Design review of the part built by this model. Coordinates are the model's own, in mm. A direction names the side the tool comes from. Give positions to 0.01 mm unless a question says otherwise; leave off trailing zeros. Loops run counter-clockwise (first coordinate to the right, second up) from the corner with the lowest first, then second, coordinate; pieces in that order, holes last. Notation, with made-up numbers: (35, 58) -> (63, 58) arc R25 ccw to (63, 77) -> close; hole circle Ø1 at (37, 37.5). An arc over 180 degrees is marked (long way). Use a Markdown table: item, result. Add a question column.
1. Draft analysis for pull direction Z (two halves, no side actions). For faces 6 (the cylindrical face through (153.73, 74.99, -0.36)), 7 (the cylindrical face through (173.43, 54.89, 4.93)), 8 (the cylindrical face through (73.547, 25.984, -58.915)), state which applies: pulls with the +Z half, pulls with the -Z half, needs draft (parallel to the pull), parting line crosses it, or undercut.
2. For faces 1 (the cylindrical face through (117.019, 12.777, 9.145)), 2 (the cylindrical face through (117.019, 12.777, 0.855)), 3 (the flat face through (116.117, 12, 5)), 4 (the flat face through (142, 33, 0)), 5 (the cylindrical face through (73.547, 47.054, -48.879)), list the 3-axis set-ups (+Z, -Z, +X, -X, +Y, -Y) from which the entire face can be reached by the end or side of a thin tool; tool diameter is ignored.
3. To check wall thickness, follow line 1 (Y direction, x = 113.5, z = -25.5); line 2 (X direction, y = 60.5, z = -61); line 3 (Y direction, x = 78, z = -43). State the ranges of each line that lie inside material, in increasing order.
4. Add section D-D (x = 188.5). State the section outline as (y, z) points.
5. For pin 1 Ø6.5 at (x, y) = (155.62, 56.56) entering from -Z; pin 2 Ø1 at (y, z) = (67, -44.5) entering from +X; pin 3 Ø3 at (y, z) = (15.5, 4) entering from +X, all flat-tipped, find the tip position at first contact; note any pin that passes through.
6. Add section C-C (z = -15.5). State the section outline as (x, y) points, and give its area (3 significant figures).
7. Add section B-B (x = 107.5). State the section outline as (y, z) points.
8. Add section A-A (z = -40). State the section outline as (x, y) points, and give its area (3 significant figures).
```python
from build123d import *

# Parameters (mm, degrees)
SKETCH3_R           = 7.5
SKETCH3_R_2         = 2.75
BOSS_EXTRUDE1_DEPTH = 10
SKETCH4_W           = 10
SKETCH4_H           = 95
BOSS_EXTRUDE2_DEPTH = 70
SKETCH8_R           = 7.5
SKETCH8_R_2         = 2.75
CUT_EXTRUDE2_DEPTH  = 43.8
BOSS_EXTRUDE3_DEPTH = 10
FILLET1_R           = 5
SKETCH11_W          = 25
SKETCH11_H          = 25
CUT_EXTRUDE3_DEPTH  = 11
FILLET3_R           = 3


with BuildPart() as part:
    # Sketch3 → Boss-Extrude1 (new body)
    with BuildSketch(Plane.XY):
        with BuildLine():
            Line((68.617133813, 80.05993294), (163.617133813, 80.05993294))
            ThreePointArc((163.617133813, 80.05993294), (191.90140506, 68.344204188), (203.617133813, 40.05993294))
            Line((203.617133813, 40.05993294), (203.617133813, 25.05993294))
            ThreePointArc((203.617133813, 25.05993294), (191.90140506, -3.224338307), (163.617133813, -14.94006706))
            Line((163.617133813, -14.94006706), (68.617133813, -14.94006706))
            Line((68.617133813, -14.94006706), (68.617133813, 80.05993294))
        make_face()
        with Locations((163.617133813, 32.55993294)):
            Circle(SKETCH3_R, mode=Mode.SUBTRACT)
        with Locations((189.617133813, 42.55993294)):
            Circle(SKETCH3_R_2, mode=Mode.SUBTRACT)
        with Locations((155.617133813, 56.55993294)):
            Circle(SKETCH3_R_2, mode=Mode.SUBTRACT)
        with Locations((175.617133813, 56.55993294)):
            Circle(SKETCH3_R_2, mode=Mode.SUBTRACT)
        with Locations((155.617133813, 8.55993294)):
            Circle(SKETCH3_R_2, mode=Mode.SUBTRACT)
        with Locations((175.617133813, 8.55993294)):
            Circle(SKETCH3_R_2, mode=Mode.SUBTRACT)
        with Locations((189.617133813, 22.55993294)):
            Circle(SKETCH3_R_2, mode=Mode.SUBTRACT)
    extrude(amount=BOSS_EXTRUDE1_DEPTH)

    # Sketch4 → Boss-Extrude2 (add)
    with BuildSketch(Plane(origin=(0, 0, 0), x_dir=(-1, 0, 0), z_dir=(0, 0, -1))):
        with Locations((-73.617133813, 32.55993294)):
            Rectangle(SKETCH4_W, SKETCH4_H)
    extrude(amount=BOSS_EXTRUDE2_DEPTH)

    # Sketch8 → Cut-Extrude2 (cut)
    with BuildSketch(Plane.ZY.offset(-68.617133813)):
        with Locations((-40, 32.55993294)):
            Circle(SKETCH8_R)
        with Locations((-56.167891819, 25.862972874)):
            Circle(SKETCH8_R_2)
        with Locations((-56.167891819, 39.256893006)):
            Circle(SKETCH8_R_2)
        with Locations((-46.696960066, 48.727824759)):
            Circle(SKETCH8_R_2)
        with Locations((-33.303039934, 48.727824759)):
            Circle(SKETCH8_R_2)
        with Locations((-23.832108181, 39.256893006)):
            Circle(SKETCH8_R_2)
        with Locations((-23.832108181, 25.862972874)):
            Circle(SKETCH8_R_2)
        with Locations((-33.303039934, 16.392041121)):
            Circle(SKETCH8_R_2)
        with Locations((-46.696960066, 16.392041121)):
            Circle(SKETCH8_R_2)
    extrude(amount=-CUT_EXTRUDE2_DEPTH, mode=Mode.SUBTRACT)

    # Sketch9 → Boss-Extrude3 (add)
    with BuildSketch(Plane.XZ.offset(14.94006706)):
        Polygon((78.617133813, -70), (153.617133813, 0), (78.617133813, 0), align=None)
    boss_extrude3 = extrude(amount=-BOSS_EXTRUDE3_DEPTH)

    # Mirror1: Boss-Extrude3 across plane
    add(boss_extrude3.mirror(Plane(origin=(0, 32.55993294, 0), x_dir=(0, 0, 1), z_dir=(0, -1, 0))))

    # Fillet1
    fillet1_edges = [part.edges().sort_by_distance(p)[0] for p in [
        (153.617133813, -9.94006706, 0),
        (153.617133813, 75.05993294, 0),
    ]]
    fillet(fillet1_edges, radius=FILLET1_R)

    # Sketch11 → Cut-Extrude3 (cut, through all)
    with BuildSketch(Plane(origin=(0, 0, 0), x_dir=(-1, 0, 0), z_dir=(0, 0, -1))):
        with Locations((-103.617133813, 12.55993294)):
            Rectangle(SKETCH11_W, SKETCH11_H)
    extrude(amount=-CUT_EXTRUDE3_DEPTH, mode=Mode.SUBTRACT)

    # Fillet3
    fillet3_edges = [part.edges().sort_by_distance(p)[0] for p in [
        (91.117133813, 12.55993294, 10),
        (103.617133813, 0.05993294, 10),
        (116.117133813, 12.55993294, 10),
        (103.617133813, 25.05993294, 10),
        (91.117133813, 12.55993294, 0),
        (103.617133813, 25.05993294, 0),
        (116.117133813, 12.55993294, 0),
        (103.617133813, 0.05993294, 0),
    ]]
    fillet(fillet3_edges, radius=FILLET3_R)


solid = part.part
```
Taken from the geometry:
| question | item | result |
|---|---|---|
| 1 | face 6 | pulls with the -Z half |
| 1 | face 7 | needs draft |
| 1 | face 8 | undercut |
| 2 | face 1 | +Z |
| 2 | face 2 | -Z |
| 2 | face 3 | +Z, -Z |
| 2 | face 4 | -Z, +X |
| 2 | face 5 | +X, -X |
| 3 | line 1 | y = -14.94 to -4.94, 70.06 to 80.06 |
| 3 | line 2 | x = 68.62 to 78.62 |
| 3 | line 3 | y = -14.94 to 25.69, 39.43 to 80.06 |
| 4 | outline | (-6.26, 0) -> (20.05, 0) -> (20.05, 10) -> (-6.26, 10) -> close; (25.07, 0) -> (40.05, 0) -> (40.05, 10) -> (25.07, 10) -> close; (45.07, 0) -> (71.38, 0) -> (71.38, 10) -> (45.07, 10) -> close |
| 5 | pin 1 | stops at z = 0 |
| 5 | pin 2 | stops at x = 78.62 |
| 5 | pin 3 | stops at x = 202.8 |
| 6 | outline | (68.62, -14.94) -> (137.01, -14.94) -> (137.01, -4.94) -> (78.62, -4.94) -> (78.62, 70.06) -> (137.01, 70.06) -> (137.01, 80.06) -> (68.62, 80.06) -> close |
| 6 | area | 2,120 mm^2 |
| 7 | outline | (-14.94, -43.04) -> (-4.94, -43.04) -> (-4.94, 0) -> (-2.94, 0) arc R3 ccw to (0.06, 3) -> (0.06, 7) arc R3 ccw to (-2.94, 10) -> (-14.94, 10) -> close; (25.06, 3) arc R3 ccw to (28.06, 0) -> (70.06, 0) -> (70.06, -43.04) -> (80.06, -43.04) -> (80.06, 10) -> (28.06, 10) arc R3 ccw to (25.06, 7) -> close |
| 8 | outline | (68.62, -14.94) -> (110.76, -14.94) -> (110.76, -4.94) -> (78.62, -4.94) -> (78.62, 25.06) -> (68.62, 25.06) -> close; (68.62, 40.06) -> (78.62, 40.06) -> (78.62, 70.06) -> (110.76, 70.06) -> (110.76, 80.06) -> (68.62, 80.06) -> close |
| 8 | area | 1,440 mm^2 |
